For this review, take the finished solid that the model builds, in its own axes (mm). A direction names the side the tool comes from. Coordinates: 2 decimals unless noted, no trailing zeros. Write each loop counter-clockwise with the first axis right and the second up, starting at its lowest first coordinate (ties: lowest second). Pieces come first, ordered by that corner, then holes. Notation, with made-up numbers: (35, 33.5) -> (52, 33.5) arc R14 cw to (52, 44.5) -> close; hole circle Ø9 at (-2, 36). An arc over 180 degrees is marked (long way). One line per item, written item: value. Start each with the question number.
1) Add section A-A (x = 17.6). State the section outline as (y, z) points.
2) Mouldability with a two-part tool opening along Z and no side actions: class faces 1 (the flat face through (27.81, 46.71, -0.07)), 2 (the flat face through (26, 45, 5)), 3 (the flat face through (24, 45, -3.5)), 4 (the flat face through (19.596, 48.431, 0.049)) as released by +Z, released by -Z, zero draft, split by the parting line, or undercut.
3) For probe 1 along Y at (x, z) = (17.6, -4.4); probe 2 along Z at (x, y) = (35, 42.75); probe 3 along Y at (x, z) = (37, -4), list the stretches that pass through material, from the lowest coordinate up. Write a range as from..to.
4) Add section B-B (y = 46.7). State the section outline as (x, z) points, and give its area (3 significant figures).
5) For pin 1 Ø1.2 at (x, z) = (23.5, -4.5) entering from -Y; pin 2 Ø5 at (x, z) = (29, 0.5) entering from +Y, all flat-tipped, find the tip position at first contact; note any pin that passes through.
6) Add section C-C (y = 40.5). State the section outline as (x, z) points.
7) Machinability: for faces 5 (the cylindrical face through (32.805, 42.977, 4.24)), 6 (the cylindrical face through (37.4, 40.3, 4.2)), 7 (the flat face through (35.555, 43.543, 0.049)), which of the approach directions +Z, -Z, +X, -X, +Y, -Y give a long, thin tool a straight path to every point of the face, cutting with its end or side? Answer none if there is none.
8) Add section D-D (z = 4.5). State the section outline as (x, y) points, and give its area (3 significant figures).
Autodesk Inventor part; units mm, degrees
ref_plane "Work Plane1" through (36.9719, 42.3357, 5) normal (0.2928471, 0.9561593, 0) x (0.9561593, -0.2928471, 0)
ref_plane "YZ Plane" through (0, 0, 0) normal (1, 0, 0) x (0, 1, 0)
ref_plane "XZ Plane" through (0, 0, 0) normal (0, 1, 0) x (-1, 0, 0)
sketch "Sketch1" plane through (0, 0, 0) normal (0, 0, 1) x (1, 0, 0)
  circle A0 centre (17.6, 46.7) radius 1.2
  circle A1 centre (36.679, 41.3795) radius 1.3
  arc A2 (18.4785, 49.5685) -> (18.3735, 43.8014) centre (17.6, 46.7) ccw
  arc A3 (34.2538, 40.7726) -> (37.4111, 43.7699) centre (36.679, 41.3795) ccw
  line L0 (18.4785, 49.5685) -> (37.4111, 43.7699)
  line L1 (18.3735, 43.8014) -> (30.3735, 43.8014)
  arc A4 (34.2538, 40.7726) -> (30.3735, 43.8014) centre (30.3735, 39.8014) ccw
  circle A5 centre (36.679, 41.3795) radius 1.2
  point P0 (0, 0)
  dimension "d0" = 5
  dimension "d1" = 3
  dimension "d3" = 4
  dimension "d14" = 12
  dimension "d15" = 2.6
extrude "Extrusion1" add sketch "Sketch1" along normal mid plane 10 contours L0 A3 A4 L1 A2
ref_plane "Work Plane1" through (36.9719, 42.3357, 5) normal (0.2928471, 0.9561593, 0) x (0.9561593, -0.2928471, 0)
sketch "Sketch2" plane through (36.9719, 42.3357, 5) normal (0.2928471, 0.9561593, 0) x (0.9561593, -0.2928471, 0)
  line L0 (8.6668, 5) -> (-28.9168, 5)
  line L1 (-22.8007, 8.5) -> (2.5, 8.5)
  line L2 (2.5, 8.5) -> (2.5, 1.5)
  line L3 (2.5, 1.5) -> (-22.8007, 1.5)
  line L4 (-22.8007, 1.5) -> (-22.8007, 8.5)
  line L5 (2.5, 10) -> (2.5, 0)
  line L6 (-22.8007, 10) -> (-22.8007, 0)
  point P0 (-22.9531, 5)
  dimension "d7" = 7
extrude "Extrusion2" cut sketch "Sketch2" against normal through all
sketch "Sketch3" plane through (36.9719, 42.3357, 5) normal (-0.2928471, -0.9561593, 0) x (0.9561593, -0.2928471, 0)
  line L0 (-22.3987, -8.5) -> (-22.3987, -1.5)
  line L1 (-22.3987, -8.5) -> (2.2913, -8.5)
  line L2 (2.2913, -1.5) -> (2.2913, -8.5)
  line L3 (-22.3987, -1.5) -> (-18.3987, -1.5)
  line L4 (-18.3987, -1.5) -> (-18.3987, -8.5)
  line L5 (-18.3987, -8.5) -> (-22.3987, -8.5)
  line L6 (-22.3987, -8.5) -> (-22.3987, -1.5)
  line L7 (2.2913, -1.5) -> (-1.7087, -1.5)
  line L8 (-1.7087, -1.5) -> (-1.7087, -8.5)
  line L9 (-1.7087, -8.5) -> (2.2913, -8.5)
  line L10 (2.2913, -8.5) -> (2.2913, -1.5)
  point P0 (-22.9531, -5)
  dimension "d10" = 4
  dimension "d11" = 4
extrude "Extrusion3" cut sketch "Sketch3" against normal through all
properties part number "Lever for overlay hinge" material "Steel"
Numbers:
1. outline: (43.7, -5) -> (45.5, -5) -> (45.5, -3.5) -> (43.7, -3.5) -> close; (43.7, 3.5) -> (45.5, 3.5) -> (45.5, 5) -> (43.7, 5) -> close; (47.9, -5) -> (49.7, -5) -> (49.7, -3.5) -> (47.9, -3.5) -> close; (47.9, 3.5) -> (49.7, 3.5) -> (49.7, 5) -> (47.9, 5) -> close
2. face 1: zero draft
2. face 2: released by +Z
2. face 3: undercut
2. face 4: undercut
3. probe 1: 43.7..45.5, 47.9..49.7
3. probe 2: -5..-3.5, 3.5..5
3. probe 3: 38.9..40.12, 42.64..43.9
4. outline: (14.6, -5) -> (16.4, -5) -> (16.4, -3.5) -> (14.6, -3.5) -> close; (14.6, 3.5) -> (16.4, 3.5) -> (16.4, 5) -> (14.6, 5) -> close; (18.8, -5) -> (27.84, -5) -> (27.84, 5) -> (18.8, 5) -> (18.8, 3.5) -> (22.72, 3.5) -> (22.72, -3.5) -> (18.8, -3.5) -> close
4. area: 68.4 mm²
5. pin 1: y = 43.8
5. pin 2: y = 47.11
6. outline: (34.34, -5) -> (35.72, -5) -> (35.72, -3.5) -> (34.34, -3.5) -> close; (34.34, 3.5) -> (35.72, 3.5) -> (35.72, 5) -> (34.34, 5) -> close; (37.64, -5) -> (39.02, -5) -> (39.02, -3.5) -> (37.64, -3.5) -> close; (37.64, 3.5) -> (39.02, 3.5) -> (39.02, 5) -> (37.64, 5) -> close
7. face 5: +Z, -Z, -Y
7. face 6: +Z, -Z
7. face 7: +X, -Y
8. outline: (18.37, 43.8) -> (30.37, 43.8) arc R4 cw to (34.25, 40.77) arc R2.5 ccw (long way) to (37.41, 43.77) -> (18.48, 49.57) arc R3 ccw (long way) to start; hole circle Ø2.4 at (17.6, 46.7); hole circle Ø2.6 at (36.68, 41.38)
8. area: 87.4 mm²
